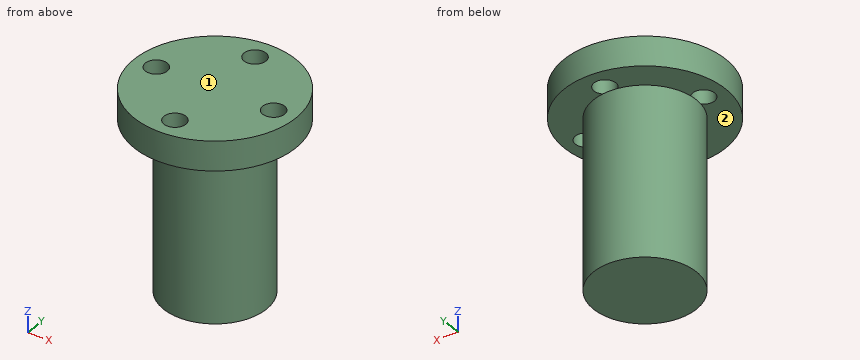
from build123d import *

# Parameters (mm, degrees)
CYLINDER004_R     = 7
CYLINDER004_DEPTH = 23
CYLINDER006_R     = 1.5
CYLINDER006_DEPTH = 20
ARRAY001_COUNT    = 4
CYLINDER005_R     = 11
CYLINDER005_DEPTH = 4


with BuildPart() as backlash_nut_cylinder:
    # Cylinder004 → Cylinder004 (new body)
    with BuildSketch(Plane.XY.offset(-23)):
        Circle(CYLINDER004_R)
    extrude(amount=CYLINDER004_DEPTH)


with BuildPart() as array001:
    # Cylinder006 → Cylinder006 (new body)
    with BuildSketch(Plane(origin=(0, -8, -5), x_dir=(1, 0, 0), z_dir=(0, 0, 1))):
        Circle(CYLINDER006_R)
    extrude(amount=CYLINDER006_DEPTH)

    # Array001: Array001 ×4 about axis
    array001_axis = Axis((0, 0, 0), (0, 0, 1))


with BuildPart() as array001_1:
    add(array001.part)
    for i in range(1, ARRAY001_COUNT):
        add(array001.part.rotate(array001_axis, i * 360 / ARRAY001_COUNT))


with BuildPart() as backlash_nut_union:
    # Cylinder005 → Cylinder005 (new body)
    with BuildSketch(Plane.XY):
        Circle(CYLINDER005_R)
    extrude(amount=CYLINDER005_DEPTH)

    # Cut: cut Array001
    add(array001_1.part, mode=Mode.SUBTRACT)

    # Fusion: union backlash nut cylinder
    add(backlash_nut_cylinder.part)


with BuildPart() as backlash_nut_union_1:
    # Fusion placement: moved
    add(backlash_nut_union.part.moved(Location((0, 0, -83))))


solid = backlash_nut_union_1.part
Work out the finished part from the listing and answer in its coordinate system (mm). Face numbers are marked on the shaded views. A direction names the side the tool comes from. Round coordinates to 2 decimals unless told otherwise and drop trailing zeros. Write each loop counter-clockwise with the first axis right and the second up, starting at its lowest first coordinate (ties: lowest second). Pieces come first, ordered by that corner, then holes. Notation, with made-up numbers: M 81.25,45.25 L 100.25,45.25 A8 cw 100.25,56.25 Z; hole C 34.25,6 d7. An arc over 180 degrees is marked long. Use a Markdown table: item, result.
1) The part is cut by section A-A on y = 0. Give the vertices of the cut face in (x, z).
Taken from the geometry:
| item | result |
|---|---|
| outline | M -11,-83 L -9.5,-83 L -9.5,-79 L -11,-79 Z; M -7,-106 L 7,-106 L 7,-83 L 6.5,-83 L 6.5,-79 L -6.5,-79 L -6.5,-83 L -7,-83 Z; M 9.5,-83 L 11,-83 L 11,-79 L 9.5,-79 Z |
2) The part is cut by section C-C on x = 8. Give the vertices of the cut face in (y, z), plus the area to 3 significant figures.
Taken from the geometry:
| item | result |
|---|---|
| outline | M -7.55,-83 L -1.5,-83 L -1.5,-79 L -7.55,-79 Z; M 1.5,-83 L 7.55,-83 L 7.55,-79 L 1.5,-79 Z |
| area | 48.4 mm2 |
3) Which of the six approach directions +Z, -Z, +X, -X, +Y, -Y give full straight-line access (tool end or side, diameter ignored) to the marked faces 1 and 2?
Taken from the geometry:
| item | result |
|---|---|
| face 1 | +Z, +X, -X, +Y, -Y |
| face 2 | -Z |
4) Consider line 1 (X direction, y = 8, z = -81.5); line 2 (Z direction, x = 7, y = -7). Determine where each line is inside the solid, lowest interval first. Write a range as [from, to].
Taken from the geometry:
| item | result |
|---|---|
| line 1 | x = [-7.55, -1.5], [1.5, 7.55] |
| line 2 | z = [-83, -79] |
5) Flat-ended cylindrical pins translate along their axes: pin 1 (1 mm diameter, centred on x = -2, z = -87, fed in from -Y); pin 2 (1.5 mm diameter, centred on y = -2.5, z = -102.5, fed in from +X); pin 3 (2.5 mm diameter, centred on x = 0, y = -8, fed in from +Z). Find the tip coordinate at first contact, or state that the pin passes through.
Taken from the geometry:
| item | result |
|---|---|
| pin 1 | stops at y = -6.84 |
| pin 2 | stops at x = 6.78 |
| pin 3 | stops at z = -83 |
